Check sheet for the modelled part. Datum: model origin and axes. Units: mm. Face numbers are marked on the shaded views. A direction names the side the tool comes from. Give positions to 0.01 mm unless a question says otherwise; leave off trailing zeros. Write each loop counter-clockwise with the first axis right and the second up, starting at its lowest first coordinate (ties: lowest second). Pieces come first, ordered by that corner, then holes. Notation, with made-up numbers: (76, -5.5) -> (132, -5.5) arc R26 cw to (132, 12.5) -> close; hole circle Ø1 at (22, 69). An arc over 180 degrees is marked (long way). Write each question's results on one line, items separated by ' | '. Start each with the question number.
```python
from build123d import *

# Parameters (mm, degrees)
SKETCH1_R             = 31.25
SKETCH1_R_2           = 29.25
SKETCH1_R_3           = 27.25
BOSS_EXTRUDE2_DEPTH   = 12
SKETCH7_R             = 16.5
SKETCH7_R_2           = 14.5
SKETCH7_R_3           = 10
BOSS_EXTRUDE6_DEPTH   = 4
SKETCH7_16_OUTSIDE_W  = 82.718
SKETCH7_16_OUTSIDE_H  = 82.718
CUT_EXTRUDE3_DEPTH    = 10
M4X0_7_TAPPED_HOLE1_D = 3.3
CUT_EXTRUDE4_START    = -10
SKETCH20_R            = 31.25
SKETCH20_R_2          = 30.25
CUT_EXTRUDE4_DEPTH    = 10


with BuildPart() as part:
    # Sketch1 → Boss-Extrude2 (new body)
    # profile 1 of 2: a face of its own
    with BuildSketch(Plane.XY):
        Circle(SKETCH1_R)
        Circle(SKETCH1_R_2, mode=Mode.SUBTRACT)
    # profile 2 of 2: a face of its own
    with BuildSketch(Plane.XY):
        Circle(SKETCH1_R_2)
        Circle(SKETCH1_R_3, mode=Mode.SUBTRACT)
    extrude(amount=BOSS_EXTRUDE2_DEPTH)



with BuildPart() as body_2:
    # Sketch7 → Boss-Extrude6 (new body)
    # profile 1 of 2: a face of its own
    with BuildSketch(Plane(origin=(0, 0, -10), x_dir=(-1, 0, 0), z_dir=(0, 0, -1))):
        Circle(SKETCH7_R)
        Circle(SKETCH7_R_2, mode=Mode.SUBTRACT)
    # profile 2 of 2: a face of its own
    with BuildSketch(Plane(origin=(0, 0, -10), x_dir=(-1, 0, 0), z_dir=(0, 0, -1))):
        Circle(SKETCH7_R_2)
        Circle(SKETCH7_R_3, mode=Mode.SUBTRACT)
    extrude(amount=-BOSS_EXTRUDE6_DEPTH)


with BuildPart() as part_1:
    add(part.part)

    add(body_2.part)  # Revolve1 merges body 2
    # Sketch10 → Revolve1 (revolve)
    with BuildSketch(Plane(origin=(0, 0, 0), x_dir=(1, 0, 0), z_dir=(0, 1, 0)), mode=Mode.PRIVATE) as revolve1_sk:
        Polygon((-16.5, 6), (-27.25, 0), (-31.25, 0), (-16.5, 10), align=None)
    revolve(revolve1_sk.sketch.rotate(Axis((0, 0, 0), (0, 0, -1)), 180), axis=Axis((0, 0, 0), (0, 0, -1)))

    # Sketch7_16 outside → Cut-Extrude3 (cut)
    with BuildSketch(Plane(origin=(0, 0, -10), x_dir=(-1, 0, 0), z_dir=(0, 0, -1))):
        Rectangle(SKETCH7_16_OUTSIDE_W, SKETCH7_16_OUTSIDE_H)
        with BuildLine():
            ThreePointArc((25.890833333, 17.499349968), (18.996047719, 9.929942094), (16.5, 0))
            ThreePointArc((16.5, 0), (18.996047719, -9.929942094), (25.890833333, -17.499349968))
            ThreePointArc((25.890833333, -17.499349968), (22.097086912, -22.097086912), (17.499349968, -25.890833333))
            ThreePointArc((17.499349968, -25.890833333), (9.929942094, -18.996047719), (0, -16.5))
            ThreePointArc((0, -16.5), (-9.929942094, -18.996047719), (-17.499349968, -25.890833333))
            ThreePointArc((-17.499349968, -25.890833333), (-22.097086912, -22.097086912), (-25.890833333, -17.499349968))
            ThreePointArc((-25.890833333, -17.499349968), (-18.996047719, -9.929942094), (-16.5, 0))
            ThreePointArc((-16.5, 0), (-18.996047719, 9.929942094), (-25.890833333, 17.499349968))
            ThreePointArc((-25.890833333, 17.499349968), (-22.097086912, 22.097086912), (-17.499349968, 25.890833333))
            ThreePointArc((-17.499349968, 25.890833333), (-9.929942094, 18.996047719), (0, 16.5))
            ThreePointArc((0, 16.5), (9.929942094, 18.996047719), (17.499349968, 25.890833333))
            ThreePointArc((17.499349968, 25.890833333), (22.097086912, 22.097086912), (25.890833333, 17.499349968))
        make_face(mode=Mode.SUBTRACT)
    extrude(amount=-CUT_EXTRUDE3_DEPTH, mode=Mode.SUBTRACT)

    # M4x0.7 Tapped Hole1 (through all)
    with Locations(Plane(origin=(0, 0, -10), x_dir=(-1, 0, 0), z_dir=(0, 0, -1))):
        with Locations((-8.838834765, 8.838834765), (8.838834765, 8.838834765), (8.838834765, -8.838834765), (-8.838834765, -8.838834765)):
            Hole(M4X0_7_TAPPED_HOLE1_D / 2)

    # Sketch20 → Cut-Extrude4 (cut)
    with BuildSketch(Plane.XY.offset(12).offset(CUT_EXTRUDE4_START)):
        with Locations(Location((0, 0, 0), (0, 0, 145.945640774))):
            Circle(SKETCH20_R)
        Circle(SKETCH20_R_2, mode=Mode.SUBTRACT)
    extrude(amount=CUT_EXTRUDE4_DEPTH, mode=Mode.SUBTRACT)


solid = part_1.part
```
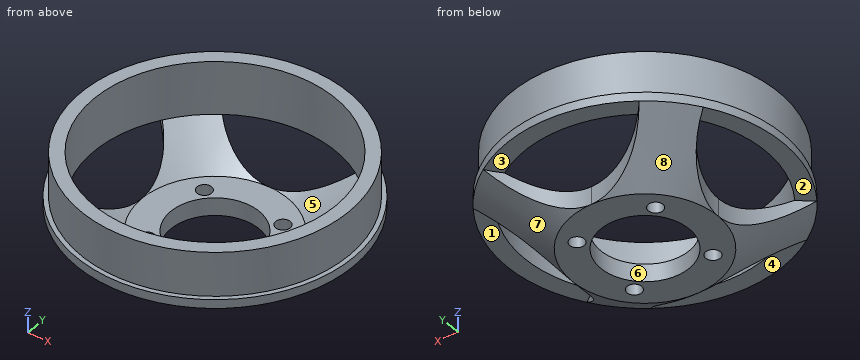
Item 1: Section check A-A on y = 2. Count the separate pieces of the cut face and the enclosed holes in it, then the cut area to 3 significant figures.
Item 2: Mould release check, pull along X, two halves, no side actions. Record for the marked faces 6, 7 and 8: pulls with the +X half, pulls with the -X half, needs draft (parallel to the pull), parting line crosses it, or undercut.
Item 3: Section check B-B on z = 8. Record the boundary of the cut face in (x, y).
Item 4: Set-up check for the marked faces 1, 2, 3, 4 and 5: record each of +Z, -Z, +X, -X, +Y, -Y from which the full face is reachable in a straight line by a thin tool's end or side.
Item 5: Thickness scan on probe 1 along Y at (x, z) = (8, -7); probe 2 along Z at (x, y) = (-3, -10); probe 3 along X at (y, z) = (20, 3). Record the ranges inside material, lowest first. Write a range as from..to.
Item 6: Depth check by flat-ended pin: pin 1 Ø9.5 at (x, y) = (2.5, -27) entering from -Z; pin 2 Ø3 at (x, y) = (-21.5, -12.5) entering from -Z; pin 3 Ø6 at (x, y) = (-14.5, -18) entering from +Z. Enter the tip coordinate at first touch or a pass-through.
Check sheet entries:
1) separate pieces: 4 | enclosed holes: 0 | area: 131 mm^2
2) face 6: undercut | face 7: pulls with the +X half | face 8: pulls with the -X half
3) outline: circle Ø60.5 at (0, 0); hole circle Ø54.5 at (0, 0)
4) face 1: -Z, +X | face 2: -Z, -X | face 3: -Z, +Y | face 4: -Z, -Y | face 5: +Z
5) probe 1: y = -18.08..-10.26, -7.42..-6, 6..7.42, 10.26..18.08 | probe 2: z = -10..-6 | probe 3: x = -22.69..-18.51, 18.51..22.69
6) pin 1: stops at z = 0 | pin 2: stops at z = -5.34 | pin 3: stops at z = -0.63
